Verification items for the finished model (mm, model axes). A direction names the side the tool comes from. Coordinates: 2 decimals unless noted, no trailing zeros. Write each loop counter-clockwise with the first axis right and the second up, starting at its lowest first coordinate (ties: lowest second). Pieces come first, ordered by that corner, then holes. Notation, with made-up numbers: M 12,-1 L 45,-1 A21 ccw 45,16 Z; hole C -14.5,47.25 d2. An arc over 180 degrees is marked long. Answer in a Markdown table with one row per item.
Autodesk Inventor part; units mm, degrees
ref_plane "Work Plane1" through (29, 0, 0) normal (0, -1, 0) x (1, 0, 0)
ref_plane "YZ Plane" through (0, 0, 0) normal (1, 0, 0) x (0, 1, 0)
ref_plane "XZ Plane" through (0, 0, 0) normal (0, 1, 0) x (-1, 0, 0)
sketch "Skizze1" plane through (0, 0, 0) normal (0, 0, 1) x (1, 0, 0)
  line L0 (-0.8667, 0) -> (12, 0)
  line L1 (12, 0) -> (12, 1.5)
  line L2 (12, 1.5) -> (1.25, 1.5)
  line L3 (1.25, 1.5) -> (0.9432, 1.5)
  line L4 (0.9432, 1.5) -> (0, 1.5)
  line L5 (0, 1.5) -> (0, 2.75)
  line L6 (0, 2.75) -> (-3, 2.75)
  line L7 (-3, 2.75) -> (-3, 1.4434)
  line L8 (-3, 1.4434) -> (-1.7, 1.4434)
  line L9 (-1.7, 1.4434) -> (-0.8667, 0)
  line L10 (-6, 0) -> (15, 0)
  line L11 (0, -0.55) -> (0, 3.3)
  line L12 (1.25, 1.5) -> (0, 1.5) construction
  dimension "d1" = 10.75
  dimension "d2" = 0.3068
  dimension "d3" = 3
  dimension "d4" = 1.3
  dimension "d5" = 60
  dimension "d6" = 3
  dimension "d7" = 3
  dimension "d8" = 2.8868
  dimension "d9" = 5.5
  dimension "d26" = 12
revolve "Körper" add sketch "Skizze1" angle 360 about axis through (-0.8667, 0, 0) along (1, 0, 0)
sketch "Skizze2" plane through (-3, 0, 0) normal (-1, 0, 0) x (0, 0, 1)
  circle A0 centre (0, 0) radius 1.4434
  line L0 (0, -3.85) -> (0, 3.85)
  line L1 (-3.85, 0) -> (3.85, 0)
  line L2 (1.4434, 0) -> (0.7217, -1.25)
  line L3 (0.7217, -1.25) -> (-0.7217, -1.25)
  line L4 (-0.7217, -1.25) -> (-1.4434, 0)
  line L5 (-1.4434, 0) -> (-0.7217, 1.25)
  line L6 (-0.7217, 1.25) -> (0.7217, 1.25)
  line L7 (0.7217, 1.25) -> (1.4434, 0)
  point P0 (0, 0)
extrude "Loch" add sketch "Skizze2" against normal up to next contours L7 A0 | A0 L2 | L6 L0 A0 | A0 L0 L3 | L0 L6 A0 | A0 L3 L0 | L4 A0 | A0 L5
fillet "Rundung1" radius 0.3 1 edges at (-3, -2.75, 0)
thread "Gewinde"
chamfer "Fase1" distance 0.3067 distance2 0.3067 1 edges at (12, -1.5, 0) measured on face at (12, -0.6587, -0.1791)
ref_plane "Work Plane1" through (29, 0, 0) normal (0, -1, 0) x (1, 0, 0)
fillet "Fillet2" radius 0.1 1 edges at (0, -1.5, 0)
sketch "Skizze4" plane through (12, 0, 0) normal (1, 0, 0) x (0, 0, -1)
  point P0 (0, 0)
equation "\"d1\" = GEL"
equation "\"d3\" = KOH"
equation "\"d4\" = INTI"
equation "\"d6\" = GD"
equation "\"d7\" = BDM"
equation "\"d8\" = 1.1547 * SW"
equation "\"d9\" = KOD"
equation "\"d26\" = NLG"
equation "\"d30\" = R"
equation "\"d17\" = RR"
equation "\"d13\" = GEL"
equation "\"d15\" = -0.5 * SPD + 0.5 * GD"
equation "\"d16\" = GUL"
equation "\"GD\" = NND"
equation "\"NLG\" = 12"
equation "\"GEL\" = 10.75"
equation "\"KOD\" = 5.5"
equation "\"KOH\" = 3"
equation "\"INTI\" = 1.3"
equation "\"GAL\" = 0.61345 * PTC"
equation "\"GUL\" = 0.61345 * PTC"
equation "\"BDM\" = NND"
equation "\"SW\" = 2.5"
equation "\"RR\" = 0.3"
equation "\"SPD\" = NND - 1.2269 * PTC"
equation "\"R\" = 0.1"
equation "\"TOA\" = 30deg"
equation "\"GD1\" = THREADDIA - 1.2269 * PTC"
equation "\"THREADDIA\" = 3"
equation "\"FAWI\" = 45deg"
equation "\"ANG\" = 120deg"
equation "\"PTC\" = 0.5"
equation "\"NND\" = 3"
equation "\"E0\" = 1.155 * SW"
properties part number "DIN 912 - M3 x 12" material "Stahl, weich"
1) Thickness scan on L1, parallel to X at y = 2.35, z = -0.65; L2, parallel to Y at x = -1.5, z = 0.4; L3, parallel to Z at x = -1.5, y = -0.55. Record the ranges inside material, lowest first. Write a range as [from, to].
Response values:
| item | result |
|---|---|
| L1 | x = [-3, 0] |
| L2 | y = [-2.72, -1.02], [1.02, 2.72] |
| L3 | z = [-2.69, -0.95], [0.95, 2.69] |
2) Depth check by flat-ended pin: pin 1 (2 mm diameter, centred on x = 3.5, z = -1.5, fed in from -Y). Enter the tip coordinate at first touch or a pass-through.
Response values:
| item | result |
|---|---|
| pin 1 | stops at y = -1.41 |
3) Tool access check on faces 1 (the face through (5.82, -1.5, -0.07)), 2 (the face through (-1.369, -0.596, 2.685)), 3 (the face through (-2.3, 0.63, 1.08)). Record the directions out of +Z, -Z, +X, -X, +Y, -Y that give a thin tool (end or side, any length) a straight path to the whole face; none if there is none.
Response values:
| item | result |
|---|---|
| face 1 | +X |
| face 2 | +X, -X |
| face 3 | -X |
4) Sectioned sample at A-A (x = 2.5). Record the cut outline in (y, z).
Response values:
| item | result |
|---|---|
| outline | C 0,0 d3 |
